For this review, use the dimensioned drawing (mm, ordinates from the lowest corner) and the shaded views. A direction names the side the tool comes from. Give positions to 0.01 mm unless a question says otherwise; leave off trailing zeros. Loops run counter-clockwise (first coordinate to the right, second up) from the corner with the lowest first, then second, coordinate; pieces in that order, holes last. Notation, with made-up numbers: M 82,-33.5 L 132,-33.5 A18 cw 132,-12.5 Z; hole C 2,-10.5 d8. An arc over 180 degrees is marked long. Return JSON: item names as keys, results as strings.
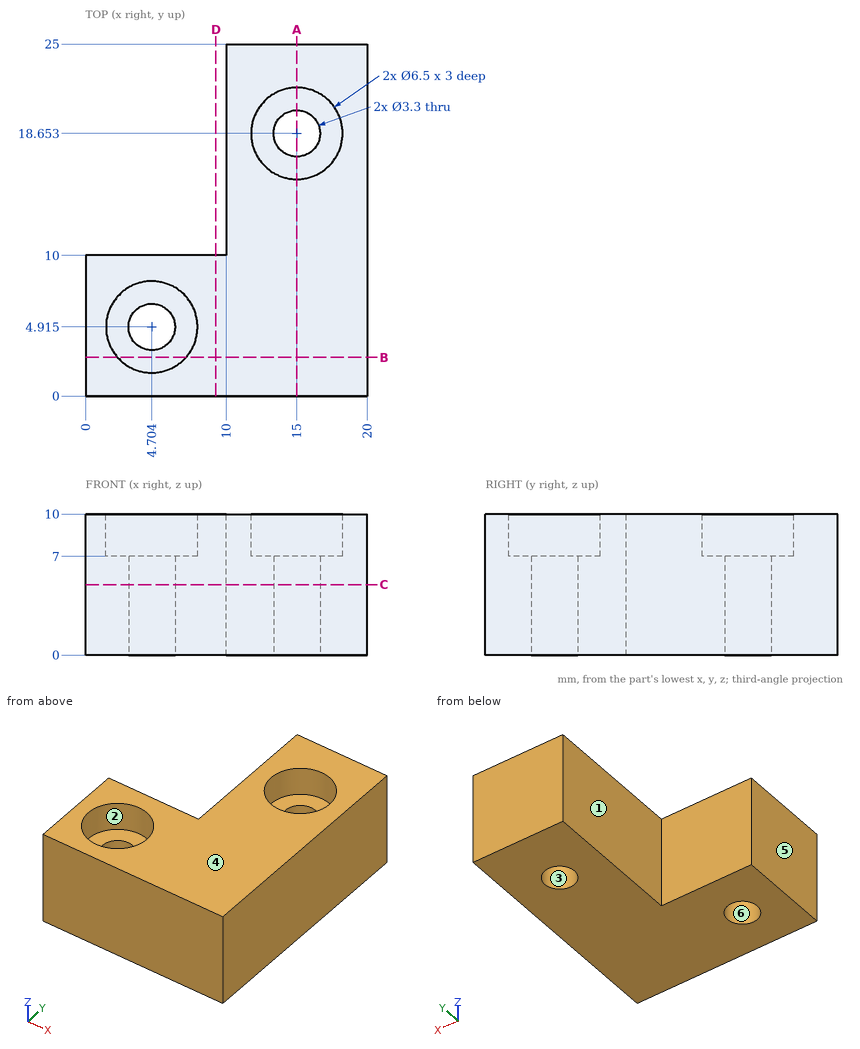
1) Wall thickness on L1, parallel to Y at x = 4.75, z = 5.75 (1 decimal); L2, parallel to Y at x = 15, z = 8; L3, parallel to X at y = 12.25, z = 1.75: over which ranges is each line inside the solid? List them lowest first. Write a range as from..to.
From the geometry:
{"L1": "0..3.3, 6.6..10", "L2": "0..15.4, 21.9..25", "L3": "10..20"}
2) The part is to be moulded in two halves that separate along X. For the marked faces 4, 5 and 6, say which applies: released by +X, released by -X, zero draft, split by the parting line, or undercut.
From the geometry:
{"face 4": "zero draft", "face 5": "released by -X", "face 6": "undercut"}
3) Consider section D-D on x = 9.25. Write out the cut boundary in (y, z), then the cut area to 3 significant figures.
From the geometry:
{"outline": "M 0,0 L 10,0 L 10,10 L 0,10 Z", "area": "100 mm²"}
4) Insertion check: pin 1 (5 mm diameter, centred on y = 21.5, z = 5.5, fed in from -X); pin 2 (6 mm diameter, centred on x = 4.7, y = 4.91, fed in from +Z); pin 3 (4 mm diameter, centred on x = 2.5, z = 1, fed in from +Y). Each pin has a flat end and moves straight along its axis. Give the tip position at first contact, or say it passes through.
From the geometry:
{"pin 1": "x = 10", "pin 2": "z = 7", "pin 3": "y = 10"}
5) Tool access review of the marked faces 1, 2 and 3: name each direction out of +Z, -Z, +X, -X, +Y, -Y from which nothing blocks a thin tool from reaching the whole face with its end or side.
From the geometry:
{"face 1": "+Z, -Z, -X, +Y", "face 2": "+Z", "face 3": "+Z, -Z"}
6) Consider section A-A on x = 15. Write out the cut boundary in (y, z).
From the geometry:
{"outline": "M 0,0 L 17,0 L 17,7 L 15.4,7 L 15.4,10 L 0,10 Z; M 20.3,0 L 25,0 L 25,10 L 21.9,10 L 21.9,7 L 20.3,7 Z"}
7) Consider section B-B on y = 2.75. Write out the cut boundary in (x, z), then the cut area to 3 significant figures.
From the geometry:
{"outline": "M 0,0 L 20,0 L 20,10 L 7.13,10 L 7.13,7 L 2.28,7 L 2.28,10 L 0,10 Z", "area": "185 mm²"}
8) Consider section C-C on z = 5. Count the separate pieces of the cut face and the enclosed holes in it, then the cut area to 3 significant figures.
From the geometry:
{"separate pieces": "1", "enclosed holes": "2", "area": "333 mm²"}
